```python
from build123d import *

# Parameters (mm, degrees)
F0_W      = 139.7
F0_H      = 241.3
F1_DEPTH  = 12.7
F3_D      = 14.2875
F4_W      = 228.6
F4_H      = 12.7
F5_DEPTH  = 222.25
F7_DEPTH  = 228.601
F9_DEPTH  = 228.601
F10_W     = 139.7
F10_H     = 203.2
F11_DEPTH = 12.7
F13_DEPTH = 25.4


with BuildPart() as f1:
    # F0 (on Top) → F1 (new body)
    with BuildSketch(Plane.XY):
        Rectangle(F0_W, F0_H)
    extrude(amount=F1_DEPTH)

    # F3 (through all)
    with Locations(Plane.XY.offset(12.7)):
        with Locations((-50.8, 63.5), (50.8, 63.5), (50.8, -63.5), (-50.8, -63.5)):
            Hole(F3_D / 2)

    # F4 (on face) → F5 (join)
    with BuildSketch(Plane.XY.offset(12.7)):
        with Locations((-44.45, -101.6)):
            Rectangle(F4_W, F4_H)
        with Locations((-44.45, 101.6)):
            Rectangle(F4_W, F4_H)
    extrude(amount=F5_DEPTH)

    # F6 (on face) → F7 (cut, through all)
    with BuildSketch(Plane.XZ.offset(107.95)):
        Polygon((-158.75, 12.7), (-69.85, 12.7), (-69.85, 63.5), (-158.75, 234.95), align=None)
    extrude(amount=-F7_DEPTH, mode=Mode.SUBTRACT)

    # F8 (on face) → F9 (cut, through all)
    with BuildSketch(Plane.XZ.offset(107.95)):
        Polygon((69.85, 234.95), (-19.05, 234.95), (69.85, 12.7), align=None)
    extrude(amount=-F9_DEPTH, mode=Mode.SUBTRACT)

    # F10 (on face) → F11 (join)
    with BuildSketch(Plane.XY.offset(234.95)):
        with Locations((-88.9, 0)):
            Rectangle(F10_W, F10_H)
    extrude(amount=F11_DEPTH)

    # F12 (on face) → F13 (cut)
    with BuildSketch(Plane.XY.offset(247.65)):
        with BuildLine():
            ThreePointArc((-134.112, -57.912), (-139.7, -63.5), (-134.112, -69.088))
            Line((-134.112, -69.088), (-119.888, -69.088))
            ThreePointArc((-119.888, -69.088), (-114.3, -63.5), (-119.888, -57.912))
            Line((-119.888, -57.912), (-134.112, -57.912))
        make_face()
        with BuildLine():
            Line((-57.912, -69.088), (-43.688, -69.088))
            ThreePointArc((-43.688, -69.088), (-38.1, -63.5), (-43.688, -57.912))
            Line((-43.688, -57.912), (-57.912, -57.912))
            ThreePointArc((-57.912, -57.912), (-63.5, -63.5), (-57.912, -69.088))
        make_face()
        with BuildLine():
            Line((-57.912, 57.912), (-43.688, 57.912))
            ThreePointArc((-43.688, 57.912), (-38.1, 63.5), (-43.688, 69.088))
            Line((-43.688, 69.088), (-57.912, 69.088))
            ThreePointArc((-57.912, 69.088), (-63.5, 63.5), (-57.912, 57.912))
        make_face()
        with BuildLine():
            Line((-119.888, 69.088), (-134.112, 69.088))
            ThreePointArc((-134.112, 69.088), (-139.7, 63.5), (-134.112, 57.912))
            Line((-134.112, 57.912), (-119.888, 57.912))
            ThreePointArc((-119.888, 57.912), (-114.3, 63.5), (-119.888, 69.088))
        make_face()
    extrude(amount=-F13_DEPTH, mode=Mode.SUBTRACT)


solid = f1.part
```
Geometry check sheet. Reference: the model listing, model coordinates, mm. A direction names the side the tool comes from. Coordinates: 2 decimals unless noted, no trailing zeros. Write each loop counter-clockwise with the first axis right and the second up, starting at its lowest first coordinate (ties: lowest second). Pieces come first, ordered by that corner, then holes. Notation, with made-up numbers: M 48,41 L 62,41 A9 cw 62,48 Z; hole C -15,-34 d11. An arc over 180 degrees is marked long. Use one line per item in the form item = value. Start each with the question number.
1) Section check D-D on x = -4. Enter the section's corners in (y, z) (3 decimals), and give its area (3 significant figures).
2) Release check for a two-part mould opening along Y. For faces 4 (the cylindrical face through (-49.251, 56.526, 6.261)), 5 (the flat face through (-127, -57.912, 241)), 6 (the flat face through (-90, -101.6, 241)), 7 (the flat face through (-158.75, -1, 241)) record: pulls with the +Y half, pulls with the -Y half, needs draft (parallel to the pull), parting line crosses it, or undercut.
3) Section check C-C on z = 104. Enter the section's corners in (x, y), and give its area (3 significant figures).
4) Section check A-A on x = -50.8. State how many separate pieces and enclosed holes the cut face has, and give its area (3 significant figures).
5) Section check B-B on y = -63.5. Enter the section's corners in (x, z), and give its area (3 significant figures).
6) Thickness scan on probe 1 along X at (y, z) = (-63, 9); probe 2 along Y at (x, z) = (50.8, 4.5); probe 3 along Y at (x, z) = (-37.5, 166.5). Record the ranges inside material, lowest first. Write a range as from..to.
7) Set-up check for faces 1 (the cylindrical face through (-139.7, -63.4, 241.4)), 2 (the cylindrical face through (-38.1, -63.6, 241.4)), 3 (the flat face through (-90, -105, 234.95)): record each of +Z, -Z, +X, -X, +Y, -Y from which the full face is reachable in a straight line by a thin tool's end or side.
8) Go/stop test with flat-tipped pins: pin 1 Ø1 at (x, y) = (-120.5, 38.5) entering from -Z; pin 2 Ø3 at (x, y) = (-62, -105.5) entering from +Z; pin 3 Ø8 at (x, y) = (-10, 31.5) entering from +Z. Record where each tip stops, or that it passes through.
Responses:
q1.outline = M -120.65,0 L 120.65,0 L 120.65,12.7 L 107.95,12.7 L 107.95,197.325 L 95.25,197.325 L 95.25,12.7 L -95.25,12.7 L -95.25,197.325 L -107.95,197.325 L -107.95,12.7 L -120.65,12.7 Z
q1.area = 7,750 mm2
q2.face_4 = undercut
q2.face_5 = undercut
q2.face_6 = pulls with the -Y half
q2.face_7 = needs draft
q3.outline = M -90.85,-107.95 L 33.33,-107.95 L 33.33,-95.25 L -90.85,-95.25 Z; M -90.85,95.25 L 33.33,95.25 L 33.33,107.95 L -90.85,107.95 Z
q3.area = 3,150 mm2
q4.separate_pieces = 4
q4.enclosed_holes = 0
q4.area = 10,600 mm2
q5.outline = M -158.75,234.95 L -139.7,234.95 L -139.7,247.65 L -158.75,247.65 Z; M -114.3,234.95 L -63.5,234.95 L -63.5,247.65 L -114.3,247.65 Z; M -69.85,0 L -57.94,0 L -57.94,12.7 L -69.85,12.7 Z; M -43.66,0 L 43.66,0 L 43.66,12.7 L -43.66,12.7 Z; M -38.1,234.95 L -19.05,234.95 L -19.05,247.65 L -38.1,247.65 Z; M 57.94,0 L 69.85,0 L 69.85,12.7 L 57.94,12.7 Z
q5.area = 2,540 mm2
q6.probe_1 = -69.85..-57.93, -43.67..43.67, 57.93..69.85
q6.probe_2 = -120.65..-70.64, -56.36..56.36, 70.64..120.65
q6.probe_3 = -107.95..-95.25, 95.25..107.95
q7.face_1 = +Z, -Z
q7.face_2 = +Z
q7.face_3 = +Z, +X, -X, -Y
q8.pin_1 = 234.95
q8.pin_2 = 234.95
q8.pin_3 = 12.7
